from build123d import *

# Parameters (mm, degrees)
F1_DEPTH = 18.6944


with BuildPart() as f1:
    # F0 (on Top) → F1 (new body)
    with BuildSketch(Plane.XY):
        Polygon((43.140249, 437.981573), (-312.459751, -70.018427), (-287.059751, -70.018427), (-287.059751, -88.712827), (-210.859751, -88.712827), (-210.859751, -70.018427), (-58.459751, -70.018427), (-58.459751, -88.712827), (17.740249, -88.712827), (17.740249, -70.018427), (43.140249, -70.018427), align=None)
        Polygon((-159.476273, -10.720534), (-174.791323, 0), (-131.093492, 62.425472), (-115.778443, 51.704938), align=None, mode=Mode.SUBTRACT)
        Polygon((0, 249.701889), (15.315049, 238.981355), (-28.382781, 176.555883), (-43.697831, 187.276417), align=None, mode=Mode.SUBTRACT)
    extrude(amount=F1_DEPTH)


solid = f1.part
Can you work these out from the model? Positions are in its coordinate system, mm. A direction names the side the tool comes from. Round coordinates to 2 decimals unless told otherwise and drop trailing zeros. Loops run counter-clockwise (first coordinate to the right, second up) from the corner with the lowest first, then second, coordinate; pieces in that order, holes last. Notation, with made-up numbers: (39.5, 36) - (88.5, 36) arc R18 ccw to (88.5, 52) - close; hole circle Ø9 at (35, -33.75). An arc over 180 degrees is marked (long way). Write item = value, one per line. Start each with the question number.
(1) If we section it at D-D (x = -253.5): Please give me the cut outline in (y, z), and give its area (3 significant figures).
(2) If we section it at C-C (z = 6.5): Please give me the cut outline in (x, y), and give its area (3 significant figures).
(3) If we section it at A-A (x = -146): Please give me the cut outline in (y, z), and give its area (3 significant figures).
(4) For faces 1 (the face through (-21, -88.713, 9)), 2 (the face through (-167.027, -5.435, 9.216)), 3 (the face through (-300, -70.018, 9)), 4 (the face through (30, -70.018, 9)), 5 (the face through (-210.86, -79, 9)), which set-ups out of +Z, -Z, +X, -X, +Y, -Y let a thin tool reach every point of the face, with its end or its side?
(5) If I drill on probe 1 along X at (y, z) = (30.5, 5); probe 2 along X at (y, z) = (200, 6.25); probe 3 along Y at (x, z) = (-129.5, 6.5), over which ranges is the centre line in solid material (lowest first)? Write a range as [from, to].
(6) For P1, Ø9.5, axis at x = -294, z = 13.5, coming from the -Y side; P2, Ø1.5, axis at x = -148.5, z = 6.5, coming from the +Y side; P3, Ø5.5, axis at y = -82.5, z = 9, coming from the -X side, each with a flat end and sliding along its axis, tell me the tip position at first contact or that it passes through.
(7) If we section it at B-B (y = 208): Please give me the cut outline in (x, z), and give its area (3 significant figures).
Ans:
q1.outline = (-88.71, 0) - (14.21, 0) - (14.21, 18.69) - (-88.71, 18.69) - close
q1.area = 1,920 mm²
q2.outline = (-312.46, -70.02) - (-287.06, -70.02) - (-287.06, -88.71) - (-210.86, -88.71) - (-210.86, -70.02) - (-58.46, -70.02) - (-58.46, -88.71) - (17.74, -88.71) - (17.74, -70.02) - (43.14, -70.02) - (43.14, 437.98) - close; hole (-174.79, 0) - (-159.48, -10.72) - (-115.78, 51.7) - (-131.09, 62.43) - close; hole (-43.7, 187.28) - (-28.38, 176.56) - (15.32, 238.98) - (0, 249.7) - close
q2.area = 90,300 mm²
q3.outline = (-70.02, 0) - (8.53, 0) - (8.53, 18.69) - (-70.02, 18.69) - close; (41.13, 0) - (167.78, 0) - (167.78, 18.69) - (41.13, 18.69) - close
q3.area = 3,840 mm²
q4.face_1 = +Z, -Z, +X, -X, -Y
q4.face_2 = +Z, -Z
q4.face_3 = +Z, -Z, -X, -Y
q4.face_4 = +Z, -Z, +X, -Y
q4.face_5 = +Z, -Z, -Y
q5.probe_1 = [-242.1, -153.44], [-130.62, 43.14]
q5.probe_2 = [-123.45, -34.79], [-11.97, 43.14]
q5.probe_3 = [-70.02, 32.1], [61.31, 191.35]
q6.P1 = -70.02
q6.P2 = 165.28
q6.P3 = -287.06
q7.outline = (-117.85, 0) - (-29.19, 0) - (-29.19, 18.69) - (-117.85, 18.69) - close; (-6.37, 0) - (43.14, 0) - (43.14, 18.69) - (-6.37, 18.69) - close
q7.area = 2,580 mm²
